The model under review builds one solid part; all positions refer to its coordinate system, in mm. Face numbers are marked on the shaded views. Coordinates: 2 decimals unless noted, no trailing zeros. Write each loop counter-clockwise with the first axis right and the second up, starting at its lowest first coordinate (ties: lowest second). Pieces come first, ordered by that corner, then holes.
```python
from build123d import *

# Parameters (mm, degrees)
F0_R     = 5.75
F0_R_2   = 3.85
F0_R_3   = 3.6
F1_DEPTH = 30
F2_DEPTH = 15
F3_START = 15
F3_DEPTH = 15


# Not quite as in the source:
# - a fillet or chamfer that OpenCascade refuses, or shapes differently, is made with other operations: its cross-section is extruded or revolved along the edge and cut away or added
# - a feature names something its author has since deleted; it is built from what else it names


with BuildPart() as f1:
    # F0 (on Top) → F1 (new body)
    with BuildSketch(Plane.XY):
        Circle(F0_R)
        Circle(F0_R_2, mode=Mode.SUBTRACT)
        Circle(F0_R_2)
        Circle(F0_R_3, mode=Mode.SUBTRACT)
        Circle(F0_R_3)
    extrude(amount=F1_DEPTH)

    # F0 (on Top) → F2 (cut)
    with BuildSketch(Plane.XY):
        Circle(F0_R_3)
    extrude(amount=F2_DEPTH, mode=Mode.SUBTRACT)

    # F0 (on Top) → F3 (cut)
    with BuildSketch(Plane.XY.offset(F3_START)):
        Circle(F0_R_2)
        Circle(F0_R_3, mode=Mode.SUBTRACT)
        Circle(F0_R_3)
    extrude(amount=F3_DEPTH, mode=Mode.SUBTRACT)

    # F4: fillet of radius 2 on 2 edges, made by hand

    # F4_s1 → F4_t2 (revolve, cut)
    with BuildSketch(Plane.XZ):
        with BuildLine():
            ThreePointArc((5.75, 28.0025015645), (5.1991376746, 29.3809064397), (3.85, 30))
            Line((3.85, 30), (5.75, 30))
            Line((5.75, 30), (5.75, 28.0025015645))
        make_face()
    revolve(axis=Axis((0, 0, 30), (0, 0, 1)), mode=Mode.SUBTRACT)

    # F4_s3 → F4_t4 (revolve, cut)
    with BuildSketch(Plane.XZ):
        with BuildLine():
            ThreePointArc((5.75, 2), (5.1642135624, 0.5857864376), (3.75, 0))
            Line((3.75, 0), (5.75, 0))
            Line((5.75, 0), (5.75, 2))
        make_face()
    revolve(axis=Axis((0, 0, 0), (0, 0, 1)), mode=Mode.SUBTRACT)


solid = f1.part
```
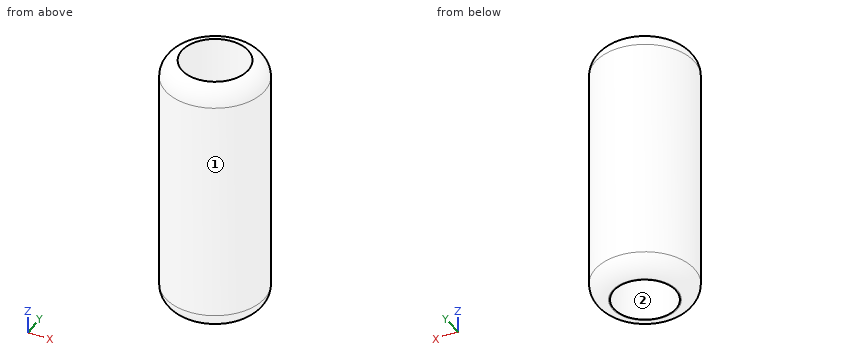
Item 1: To check wall thickness, follow line 1 along Y through (x, z) = (0, 6.75); line 2 along X through (y, z) = (0.25, 11.25); line 3 along Y through (x, z) = (-2, 15.5). State the ranges of each line that lie inside material, in increasing order.
Solved:
line 1: y = -5.75 to -3.6, 3.6 to 5.75
line 2: x = -5.74 to -3.59, 3.59 to 5.74
line 3: y = -5.39 to -3.29, 3.29 to 5.39
Item 2: Take a section at C-C, the plane z = 16. Write out the cut boundary in (x, y).
Solved:
outline: circle Ø11.5 at (0, 0); hole circle Ø7.7 at (0, 0)
Item 3: For pin 1 (5 mm diameter, centred on x = 3.5, y = 0, fed in from +Z); pin 2 (4 mm diameter, centred on x = 0.5, y = 1, fed in from +Z) (3 decimals), all flat-tipped, find the tip position at first contact; note any pin that passes through.
Solved:
pin 1: stops at z = 30
pin 2: passes through
Item 4: Mouldability with a two-part tool opening along X and no side actions: class the marked faces 1 and 2 as pulls with the +X half, pulls with the -X half, needs draft (parallel to the pull), parting line crosses it, or undercut.
Solved:
face 1: parting line crosses it
face 2: undercut
Item 5: Take a section at A-A, the plane y = 0. Write out the cut boundary in (x, z), plus the area to 3 significant figures.
Solved:
outline: (-5.75, 2) arc R2 ccw to (-3.75, 0) - (-3.6, 0) - (-3.6, 15) - (-3.85, 15) - (-3.85, 30) arc R2 ccw to (-5.75, 28) - close; (3.6, 0) - (3.75, 0) arc R2 ccw to (5.75, 2) - (5.75, 28) arc R2 ccw to (3.85, 30) - (3.85, 15) - (3.6, 15) - close
area: 118 mm2
